Verification items for the finished model (mm, model axes). Round coordinates to 2 decimals unless told otherwise and drop trailing zeros. Loops run counter-clockwise (first coordinate to the right, second up) from the corner with the lowest first, then second, coordinate; pieces in that order, holes last. Notation, with made-up numbers: (-15, 34.5) - (2, 34.5) arc R15 cw to (2, 50.5) - close; hole circle Ø3 at (72.5, 59.5). An arc over 180 degrees is marked (long way). Use a Markdown table: item, result. Add a question column.
```python
from build123d import *

# Parameters (mm, degrees)
SKETCH1_W           = 33.3375
SKETCH1_H           = 12.7
SKETCH1_R           = 1.5875
SKETCH1_R_2         = 2.38125
BOSS_EXTRUDE1_DEPTH = 3.175
FILLET1_R           = 3.175
CHAMFER2_SIZE       = 0.508
CHAMFER1_SIZE       = 0.254


with BuildPart() as part:
    # Sketch1 → Boss-Extrude1 (new body)
    with BuildSketch(Plane(origin=(0, 0, 0), x_dir=(1, 0, 0), z_dir=(0, 1, 0))):
        Rectangle(SKETCH1_W, SKETCH1_H)
        with Locations((-11.509375, 0)):
            Circle(SKETCH1_R, mode=Mode.SUBTRACT)
        with Locations((11.509375, 0)):
            Circle(SKETCH1_R, mode=Mode.SUBTRACT)
        Circle(SKETCH1_R_2, mode=Mode.SUBTRACT)
    extrude(amount=BOSS_EXTRUDE1_DEPTH)

    # Fillet1
    fillet1_edges = [part.edges().sort_by_distance(p)[0] for p in [
        (16.66875, 1.5875, 6.35),
        (-16.66875, 1.5875, 6.35),
        (-16.66875, 1.5875, -6.35),
        (16.66875, 1.5875, -6.35),
    ]]
    fillet(fillet1_edges, radius=FILLET1_R)

    # Chamfer2
    chamfer2_edges = [part.edges().sort_by_distance(p)[0] for p in [
        (16.66875, 0, 0),
        (16.66875, 3.175, 0),
        (0, 0, 6.35),
        (-16.66875, 0, 0),
        (0, 0, -6.35),
        (-15.73881403, 0, 5.42006403),
        (15.73881403, 0, -5.42006403),
        (-15.73881403, 0, -5.42006403),
        (15.73881403, 0, 5.42006403),
        (0, 3.175, 6.35),
        (0, 3.175, -6.35),
        (-16.66875, 3.175, 0),
        (-15.73881403, 3.175, 5.42006403),
        (15.73881403, 3.175, -5.42006403),
        (-15.73881403, 3.175, -5.42006403),
        (15.73881403, 3.175, 5.42006403),
    ]]
    chamfer(chamfer2_edges, length=CHAMFER2_SIZE)

    # Chamfer1
    chamfer1_edges = [part.edges().sort_by_distance(p)[0] for p in [
        (-13.096875, 0, 0),
        (-13.096875, 3.175, 0),
        (9.921875, 0, 0),
        (9.921875, 3.175, 0),
        (-2.38125, 0, 0),
        (-2.38125, 3.175, 0),
    ]]
    chamfer(chamfer1_edges, length=CHAMFER1_SIZE)


solid = part.part
```
Q1. Release check for a two-part mould opening along X. For faces 1 (the face through (-15.504, 3.03, 5.141)), 2 (the face through (16.669, 2, 0)), 3 (the face through (9.923, 1.569, -0.07)), 4 (the face through (-9.995, 1.569, -0.477)) record: +X half, -X half, draft (parallel to the pull), parting line (faces both ways), or undercut.
Q2. Go/stop test with a flat-tipped pin: pin 1 Ø3.5 at (x, z) = (-11.51, 0) entering from -Y. Record where the tip stops, or that it passes through.
Q3. Thickness scan on line 1 along X through (y, z) = (1.1, 0); line 2 along X through (y, z) = (0.4, -1); line 3 along Z through (x, y) = (0, 1.25). Record the ranges inside material, lowest first.
Q4. Section check A-A on x = 0. Record the cut outline in (y, z) (3 decimals), plus the area to 3 significant figures.
Q5. Section check B-B on z = 0. State how many separate pieces and enclosed holes the cut face has, plus the area to 3 significant figures.
Determined:
| question | item | result |
|---|---|---|
| 1 | face 1 | -X half |
| 1 | face 2 | +X half |
| 1 | face 3 | undercut |
| 1 | face 4 | undercut |
| 2 | pin 1 | stops at y = 0.09 |
| 3 | line 1 | x = -16.67 to -13.1, -9.92 to -2.38, 2.38 to 9.92, 13.1 to 16.67 |
| 3 | line 2 | x = -16.56 to -12.74, -10.28 to -2.16, 2.16 to 10.28, 12.74 to 16.56 |
| 3 | line 3 | z = -6.35 to -2.38, 2.38 to 6.35 |
| 4 | outline | (0, -5.842) - (0.508, -6.35) - (2.667, -6.35) - (3.175, -5.842) - (3.175, -2.635) - (2.921, -2.381) - (0.254, -2.381) - (0, -2.635) - close; (0, 2.635) - (0.254, 2.381) - (2.921, 2.381) - (3.175, 2.635) - (3.175, 5.842) - (2.667, 6.35) - (0.508, 6.35) - (0, 5.842) - close |
| 4 | area | 24.6 mm² |
| 5 | separate pieces | 4 |
| 5 | enclosed holes | 0 |
| 5 | area | 69.7 mm² |
